The model under review builds one solid part; all positions refer to its coordinate system, in mm. A direction names the side the tool comes from. Give positions to 0.01 mm unless a question says otherwise; leave off trailing zeros. Order: outer loops, then holes, each group sorted by start corner. A loop starts at its lowest first (then second) coordinate and runs counter-clockwise, first axis right, second up.
```python
from build123d import *

# Parameters (mm, degrees)
SKETCH_1_W           = 200
SKETCH_1_H           = 70
EXTRUDE_1_DEPTH      = 3
EXTRUDE_2_DEPTH      = 25
EXTRUDE_2_DEPTH_BACK = 25
SKETCH_6_W           = 30
SKETCH_6_H           = 37.527767497
CUT_EXTRUDE_4_DEPTH  = 65
SKETCH_7_R           = 35
CUT_EXTRUDE_5_DEPTH  = 4
SKETCH_8_W           = 3
SKETCH_8_H           = 40
EXTRUDE_3_DEPTH      = 65
SKETCH_9_R           = 1.5
CUT_EXTRUDE_6_DEPTH  = 4
SKETCH_11_W          = 65
SKETCH_11_H          = 20
CUT_EXTRUDE_7_DEPTH  = 4


with BuildPart() as part:
    # 草图1 → 凸台-拉伸1 (new body)
    with BuildSketch(Plane(origin=(0, 0, 0), x_dir=(1, 0, 0), z_dir=(0, 1, 0))):
        with Locations((17.295373665, 0)):
            Rectangle(SKETCH_1_W, SKETCH_1_H)
    extrude(amount=EXTRUDE_1_DEPTH)

    # 草图2 → 凸台-拉伸2 (add, two sides)
    with BuildSketch(Plane.XY) as extrude_2_sk:
        Polygon((-82.704626335, 40.527767497), (-82.704626335, 3), (-17.704626335, 3), align=None)
        with BuildLine():
            Line((117.295373665, 3), (117.295373665, 18.810437945))
            add(Edge.make_bspline(
                [(53.295373665, 3), (87.19337421, 4.102292249), (117.295373665, 18.810437945)],
                knots=[0, 0, 0, 1, 1, 1], degree=2))
            Line((53.295373665, 3), (117.295373665, 3))
        make_face()
    extrude(amount=EXTRUDE_2_DEPTH)
    extrude(extrude_2_sk.sketch, amount=-EXTRUDE_2_DEPTH_BACK)

    # 草图6 → 切除-拉伸4 (cut)
    with BuildSketch(Plane.ZY.offset(82.704626335)):
        with Locations((0, 21.763883748)):
            Rectangle(SKETCH_6_W, SKETCH_6_H)
    extrude(amount=-CUT_EXTRUDE_4_DEPTH, mode=Mode.SUBTRACT)

    # 草图7 → 切除-拉伸5 (cut, through all)
    with BuildSketch(Plane(origin=(0, 3, 0), x_dir=(1, 0, 0), z_dir=(0, 1, 0))):
        with Locations((25.295373665, 51)):
            Circle(SKETCH_7_R)
        with Locations((25.295373665, -51)):
            Circle(SKETCH_7_R)
    extrude(amount=-CUT_EXTRUDE_5_DEPTH, mode=Mode.SUBTRACT)

    # 草图8 → 凸台-拉伸3 (add)
    with BuildSketch(Plane.ZY.offset(82.704626335)):
        with Locations((36.5, 20)):
            Rectangle(SKETCH_8_W, SKETCH_8_H)
        with Locations((-36.5, 20)):
            Rectangle(SKETCH_8_W, SKETCH_8_H)
    extrude(amount=-EXTRUDE_3_DEPTH)

    # 草图9 → 切除-拉伸6 (cut, through all)
    with BuildSketch(Plane(origin=(0, 3, 0), x_dir=(1, 0, 0), z_dir=(0, 1, 0))):
        with Locations((-74.766784803, 29.860059225)):
            Circle(SKETCH_9_R)
        with Locations((-54.766784803, 29.860059225)):
            Circle(SKETCH_9_R)
        with Locations((-34.766784803, 29.860059225)):
            Circle(SKETCH_9_R)
        with Locations((-34.766784803, -29.860059225)):
            Circle(SKETCH_9_R)
        with Locations((-54.766784803, -29.860059225)):
            Circle(SKETCH_9_R)
        with Locations((-74.766784803, -29.860059225)):
            Circle(SKETCH_9_R)
        with Locations((68.031562246, 29.860059225)):
            Circle(SKETCH_9_R)
        with Locations((88.031562246, 29.860059225)):
            Circle(SKETCH_9_R)
        with Locations((108.031562246, 29.860059225)):
            Circle(SKETCH_9_R)
        with Locations((108.031562246, -29.860059225)):
            Circle(SKETCH_9_R)
        with Locations((88.031562246, -29.860059225)):
            Circle(SKETCH_9_R)
        with Locations((68.031562246, -29.860059225)):
            Circle(SKETCH_9_R)
    extrude(amount=-CUT_EXTRUDE_6_DEPTH, mode=Mode.SUBTRACT)

    # 草图11 → 切除-拉伸7 (cut, through all)
    with BuildSketch(Plane(origin=(0, 3, 0), x_dir=(1, 0, 0), z_dir=(0, 1, 0))):
        with Locations((-50.204626335, 0)):
            Rectangle(SKETCH_11_W, SKETCH_11_H)
    extrude(amount=-CUT_EXTRUDE_7_DEPTH, mode=Mode.SUBTRACT)


solid = part.part
```
Item 1: Take a section at B-B (x = -44.5). Give the boundary of the cut face in (y, z), and give its area (3 significant figures).
Values found:
outline: (0, -38) - (40, -38) - (40, -35) - (3, -35) - (3, -25) - (18.47, -25) - (18.47, -15) - (3, -15) - (3, -10) - (0, -10) - close; (0, 10) - (3, 10) - (3, 15) - (18.47, 15) - (18.47, 25) - (3, 25) - (3, 35) - (40, 35) - (40, 38) - (0, 38) - close
area: 699 mm2
Item 2: For line 1 (Z direction, x = -56.5, y = 23); line 2 (Z direction, x = -66.5, y = 34.5); line 3 (Y direction, x = 50, z = -5), list the stretches that pass through material, from the lowest coordinate up.
Values found:
line 1: z = -38 to -35, -25 to -15, 15 to 25, 35 to 38
line 2: z = -38 to -35, 35 to 38
line 3: y = 0 to 3
Item 3: Clearance check with flat-ended pins moving along their axes: pin 1 Ø2.5 at (x, z) = (-54.77, 29.86) entering from -Y; pin 2 Ø4 at (x, z) = (20.5, 13) entering from +Y; pin 3 Ø2.5 at (x, y) = (84, 1.5) entering from -Z; pin 4 Ø2.5 at (x, y) = (100.5, 1.5) entering from +Z. State where each tip first meets the part, or that it passes through.
Values found:
pin 1: passes through
pin 2: stops at y = 3
pin 3: stops at z = -35
pin 4: stops at z = 35
Item 4: Take a section at D-D (x = -68). Give the boundary of the cut face in (y, z).
Values found:
outline: (0, -38) - (40, -38) - (40, -35) - (3, -35) - (3, -25) - (32.04, -25) - (32.04, -15) - (3, -15) - (3, -10) - (0, -10) - close; (0, 10) - (3, 10) - (3, 15) - (32.04, 15) - (32.04, 25) - (3, 25) - (3, 35) - (40, 35) - (40, 38) - (0, 38) - close
Item 5: Take a section at C-C (y = 8). Give the number of separate pieces and of enclosed holes in the cut face, and give its area (3 significant figures).
Values found:
separate pieces: 5
enclosed holes: 0
area: 2,970 mm2
Item 6: For faces 5 (the flat face through (-49.75, 21.5, 20.07)), 6 (the flat face through (-58, 17, -15)), 7 (the flat face through (-65, 14, 25)), list the 3-axis set-ups (+Z, -Z, +X, -X, +Y, -Y) from which the entire face can be reached by the end or side of a thin tool; tool diameter is ignored.
Values found:
face 5: +Y
face 6: -X, +Y
face 7: +X, -X, +Y
Item 7: Take a section at A-A (y = 32). Give the boundary of the cut face in (x, z), and give its area (3 significant figures).
Values found:
outline: (-82.7, -38) - (-17.7, -38) - (-17.7, -35) - (-82.7, -35) - close; (-82.7, -25) - (-67.93, -25) - (-67.93, -15) - (-82.7, -15) - close; (-82.7, 15) - (-67.93, 15) - (-67.93, 25) - (-82.7, 25) - close; (-82.7, 35) - (-17.7, 35) - (-17.7, 38) - (-82.7, 38) - close
area: 685 mm2
Item 8: Draft analysis for pull direction Z (two halves, no side actions). For faces 1 (the flat face through (99, 9, 25)), 2 (the flat face through (16, 0, -1)), 3 (the flat face through (-58, 17, 15)), 4 (the flat face through (-51, 21, 35)), state which applies: released by +Z, released by -Z, zero draft, split by the parting line, or undercut.
Values found:
face 1: released by +Z
face 2: zero draft
face 3: undercut
face 4: undercut
